```python
from build123d import *

# Parameters (mm, degrees)
SKETCH_1_R           = 6
EXTRUDE_1_DEPTH      = 15
SKETCH_2_OUTSIDE_W   = 18.53
SKETCH_2_OUTSIDE_H   = 18.53
SKETCH_2_OUTSIDE_W_2 = 12
SKETCH_2_OUTSIDE_H_2 = 10
CUT_EXTRUDE_3_DEPTH  = 15
SKETCH_2_3_W         = 12
SKETCH_2_3_H         = 10
EXTRUDE_2_DEPTH      = 9
FILLET_1_R           = 0.5
SKETCH_4_R           = 2.5
EXTRUDE_3_DEPTH      = 2
SKETCH_5_R           = 1.5
CUT_EXTRUDE_4_DEPTH  = 28.147743921
FILLET_2_R           = 0.25
FILLET_3_R           = 0.25
SKETCH_6_R           = 1.95
SKETCH_6_R_2         = 1.5
EXTRUDE_4_DEPTH      = 0.6


with BuildPart() as part:
    # Sketch 1 → Extrude 1 (new body)
    with BuildSketch(Plane.XY):
        Circle(SKETCH_1_R)
    extrude(amount=EXTRUDE_1_DEPTH)

    # Sketch 2 outside → Cut-Extrude 3 (cut)
    with BuildSketch(Plane.XY.offset(15)):
        Rectangle(SKETCH_2_OUTSIDE_W, SKETCH_2_OUTSIDE_H)
        Rectangle(SKETCH_2_OUTSIDE_W_2, SKETCH_2_OUTSIDE_H_2, mode=Mode.SUBTRACT)
    extrude(amount=-CUT_EXTRUDE_3_DEPTH, mode=Mode.SUBTRACT)

    # Sketch 2_3 → Extrude 2 (add)
    with BuildSketch(Plane.XY.offset(15)):
        Rectangle(SKETCH_2_3_W, SKETCH_2_3_H)
    extrude(amount=EXTRUDE_2_DEPTH)

    # Fillet 1
    fillet_1_edges = [part.edges().sort_by_distance(p)[0] for p in [
        (6, 5, 19.5),
        (-6, 5, 19.5),
        (-6, -5, 19.5),
        (6, -5, 19.5),
    ]]
    fillet(fillet_1_edges, radius=FILLET_1_R)

    # Sketch 4 → Extrude 3 (add)
    with BuildSketch(Plane(origin=(0, 0, 0), x_dir=(-1, 0, 0), z_dir=(0, 0, -1))):
        with Locations(Location((0, 0, 0), (0, 0, 180))):
            Circle(SKETCH_4_R)
    extrude(amount=EXTRUDE_3_DEPTH)

    # Sketch 5 → Cut-Extrude 4 (cut, through all)
    with BuildSketch(Plane(origin=(0, 0, -2), x_dir=(-1, 0, 0), z_dir=(0, 0, -1))):
        Circle(SKETCH_5_R)
    extrude(amount=-CUT_EXTRUDE_4_DEPTH, mode=Mode.SUBTRACT)

    # Fillet 2
    fillet_2_edges = [part.edges().sort_by_distance(p)[0] for p in [
        (0, 5, 24),
        (6, 0, 24),
        (-6, 0, 24),
        (0, -5, 24),
        (5.853553391, -4.853553391, 24),
        (-5.853553391, -4.853553391, 24),
        (-5.853553391, 4.853553391, 24),
        (5.853553391, 4.853553391, 24),
    ]]
    fillet(fillet_2_edges, radius=FILLET_2_R)

    # Fillet 3
    fillet_3_edges = [part.edges().sort_by_distance(p)[0] for p in [
        (-2.5, 0, -2),
        (-2.5, 0, 0),
        (-3.31662479, -5, 7.5),
        (3.31662479, -5, 7.5),
        (3.31662479, 5, 7.5),
        (-3.31662479, 5, 7.5),
        (6, 0, 0),
        (-6, 0, 0),
        (0, -5, 0),
        (0, 5, 0),
    ]]
    fillet(fillet_3_edges, radius=FILLET_3_R)

    # Sketch 6 → Extrude 4 (add)
    with BuildSketch(Plane.XY.offset(24)):
        Circle(SKETCH_6_R)
        with Locations(Location((0, 0, 0), (0, 0, 180))):
            Circle(SKETCH_6_R_2, mode=Mode.SUBTRACT)
    extrude(amount=EXTRUDE_4_DEPTH)


solid = part.part
```
The model under review builds one solid part; all positions refer to its coordinate system, in mm. A direction names the side the tool comes from. Coordinates: 2 decimals unless noted, no trailing zeros. Order: outer loops, then holes, each group sorted by start corner. A loop starts at its lowest first (then second) coordinate and runs counter-clockwise, first axis right, second up. Notation, with made-up numbers: (84, -6.5) -> (129, -6.5) arc R14 ccw to (129, -2.5) -> close; hole circle Ø1 at (-30, 74.5). An arc over 180 degrees is marked (long way). Answer in a Markdown table with one row per item. Add a question column.
Item 1: We need section C-C on z = 16. Write out the cut boundary in (x, y).
Item 2: Mouldability with a two-part tool opening along Y and no side actions: class faces 6 (the cylindrical face through (-1.43, -0.45, 11.11)), 7 (the flat face through (6, 0, 19)), 8 (the cylindrical face through (-2.5, -0.1, -1)) as +Y half, -Y half, draft (parallel to the pull), parting line (faces both ways), or undercut.
Item 3: We need section A-A on x = 0. Write out the cut boundary in (y, z).
Item 4: To check wall thickness, follow probe 1 along Y at (x, z) = (0, 19); probe 2 along X at (y, z) = (0, 5); probe 3 along Z at (x, y) = (2.25, -3). State the ranges of each line that lie inside material, in increasing order.
Item 5: Machinability: for faces 1 (the flat face through (-5, 4, 15)), 2 (the cylindrical face through (-6, 0, 8)), 3 (the cylindrical face through (6, 0, 8)), 4 (the flat face through (-0.1, 2.2, 24)), 5 (the flat face through (5, -4, 15)), which of the approach directions +Z, -Z, +X, -X, +Y, -Y give a long, thin tool a straight path to every point of the face, cutting with its end or side? Answer none if there is none.
Item 6: We need section B-B on z = 7.5. Write out the cut boundary in (x, y).
Item 7: Clearance check with flat-ended pins moving along their axes: pin 1 (0.8 mm diameter, centred on x = -4, y = 3, fed in from -Z); pin 2 (2 mm diameter, centred on x = 4.5, y = 3, fed in from +Z). State where each tip first meets the part, or that it passes through.
Final values:
| question | item | result |
|---|---|---|
| 1 | outline | (-6, -4.5) arc R0.5 ccw to (-5.5, -5) -> (5.5, -5) arc R0.5 ccw to (6, -4.5) -> (6, 4.5) arc R0.5 ccw to (5.5, 5) -> (-5.5, 5) arc R0.5 ccw to (-6, 4.5) -> close; hole circle Ø3 at (0, 0) |
| 2 | face 6 | undercut |
| 2 | face 7 | draft |
| 2 | face 8 | parting line |
| 3 | outline | (-5, 0.25) arc R0.25 ccw to (-4.75, 0) -> (-2.75, 0) arc R0.25 cw to (-2.5, -0.25) -> (-2.5, -1.75) arc R0.25 ccw to (-2.25, -2) -> (-1.5, -2) -> (-1.5, 24.6) -> (-1.95, 24.6) -> (-1.95, 24) -> (-4.75, 24) arc R0.25 ccw to (-5, 23.75) -> close; (1.5, -2) -> (2.25, -2) arc R0.25 ccw to (2.5, -1.75) -> (2.5, -0.25) arc R0.25 cw to (2.75, 0) -> (4.75, 0) arc R0.25 ccw to (5, 0.25) -> (5, 23.75) arc R0.25 ccw to (4.75, 24) -> (1.95, 24) -> (1.95, 24.6) -> (1.5, 24.6) -> close |
| 4 | probe 1 | y = -5 to -1.5, 1.5 to 5 |
| 4 | probe 2 | x = -6 to -1.5, 1.5 to 6 |
| 4 | probe 3 | z = 0 to 24 |
| 5 | face 1 | -Z, -X, +Y |
| 5 | face 2 | -Z, -X |
| 5 | face 3 | -Z, +X |
| 5 | face 4 | +Z |
| 5 | face 5 | -Z, +X, -Y |
| 6 | outline | (-3.38, -4.96) arc R0.25 ccw to (-3.24, -5) -> (3.24, -5) arc R0.25 ccw to (3.38, -4.96) arc R6 ccw to (3.38, 4.96) arc R0.25 ccw to (3.24, 5) -> (-3.24, 5) arc R0.25 ccw to (-3.38, 4.96) arc R6 ccw to start; hole circle Ø3 at (0, 0) |
| 7 | pin 1 | stops at z = 0 |
| 7 | pin 2 | stops at z = 24 |
